Build history of the part. All positions in model axes, mm. A direction names the side the tool comes from. Coordinates: 2 decimals unless noted, no trailing zeros. Order: outer loops, then holes, each group sorted by start corner. A loop starts at its lowest first (then second) coordinate and runs counter-clockwise, first axis right, second up. Notation, with made-up numbers: M 50.5,53 L 74.5,53 A24 ccw 74.5,69 Z; hole C 15.25,61.5 d3. An arc over 180 degrees is marked long. Write item = value, one per line. Start each with the question number.
Q1. Pull direction Y, two halves, no side cores. Call faces 1 (the face through (-0.54, -2.44, -7.4)), 2 (the face through (-6.14, -3.36, -7.4)), 3 (the face through (14, 11, -15)): released by +Y, released by -Y, zero draft, split by the parting line, or undercut.
Q2. Band-saw the part on A-A on y = 0. Write the cut outline in (x, z).
Q3. Band-saw the part on D-D on y = 25.5. Write the cut outline in (x, z), plus the area to 3 significant figures.
Q4. Pin check, flat tips, straight feed: P1, Ø3, axis at y = 18.5, z = -4, coming from the +X side; P2, Ø6, axis at x = 45.5, z = -4, coming from the +Y side; P3, Ø1, axis at x = 10, z = -2, coming from the +Y side. Stop position of each tip, or through.
Q5. Band-saw the part on B-B on z = -1.25. Write the cut outline in (x, y), plus the area to 3 significant figures.
Q6. Drill centre lines: probe 1 along Y at (x, z) = (51, -9.25); probe 2 along Y at (x, z) = (0, -11.25); probe 3 along X at (y, z) = (1, -6.5). Where is each one in solid material? Low to high.
Q7. Band-saw the part on C-C on x = 45. Write the cut outline in (y, z).
Q8. 3-axis set-ups, long thin cutter, end or side, ignore diameter. For faces 4 (the face through (40, -3, -7)), 5 (the face through (29, -7, -7)): which of +Z, -Z, +X, -X, +Y, -Y reach the whole face in a straight line?
```python
from build123d import *

# Parameters (mm, degrees)
ESQUISSE1_R        = 2.5
BOSS_EXTRU_1_DEPTH = 15
CONG_1_R           = 1


with BuildPart() as part:
    # Esquisse1 → Boss.-Extru.1 (new body)
    with BuildSketch(Plane.XY):
        with BuildLine():
            Line((20, -3), (20, 47))
            Line((20, 47), (-6.004687468, 3.597739348))
            ThreePointArc((-6.004687468, 3.597739348), (-6.09032739, -3.4507843), (0, -7))
            Line((0, -7), (60, -7))
            Line((60, -7), (60, -3))
            Line((60, -3), (20, -3))
        make_face()
        Circle(ESQUISSE1_R, mode=Mode.SUBTRACT)
    extrude(amount=-BOSS_EXTRU_1_DEPTH)

    # Congé1
    cong_1_edges = [part.edges().sort_by_distance(p)[0] for p in [
        (60, -3, -7.5),
        (60, -7, -7.5),
        (20, 47, -7.5),
    ]]
    fillet(cong_1_edges, radius=CONG_1_R)


solid = part.part
```
Recorded:
q1.face_1 = undercut
q1.face_2 = split by the parting line
q1.face_3 = zero draft
q2.outline = M -7,-15 L -2.5,-15 L -2.5,0 L -7,0 Z; M 2.5,-15 L 20,-15 L 20,0 L 2.5,0 Z
q3.outline = M 7.12,-15 L 20,-15 L 20,0 L 7.12,0 Z
q3.area = 193 mm2
q4.P1 = 20
q4.P2 = -3
q4.P3 = 31.14
q5.outline = M -6,3.6 A7 ccw 0,-7 L 59,-7 A1 ccw 60,-6 L 60,-4 A1 ccw 59,-3 L 20,-3 L 20,43.39 A1 ccw 18.14,43.9 Z; hole C 0,0 d5
q5.area = 976 mm2
q6.probe_1 = -7 to -3
q6.probe_2 = -7 to -2.5, 2.5 to 13.62
q6.probe_3 = -6.93 to -2.29, 2.29 to 20
q7.outline = M -7,-15 L -3,-15 L -3,0 L -7,0 Z
q8.face_4 = +Z, -Z, +X, +Y
q8.face_5 = +Z, -Z, +X, -X, -Y
